For this review, take the finished solid that the model builds, in its own axes (mm). Coordinates: 2 decimals unless noted, no trailing zeros. Loops run counter-clockwise (first coordinate to the right, second up) from the corner with the lowest first, then second, coordinate; pieces in that order, holes last. Notation, with made-up numbers: M 59.25,79.5 L 80.25,79.5 A19 ccw 80.25,97.5 Z; hole C 28,19 d9. An arc over 180 degrees is marked long. Put each result on its own line as item: value.
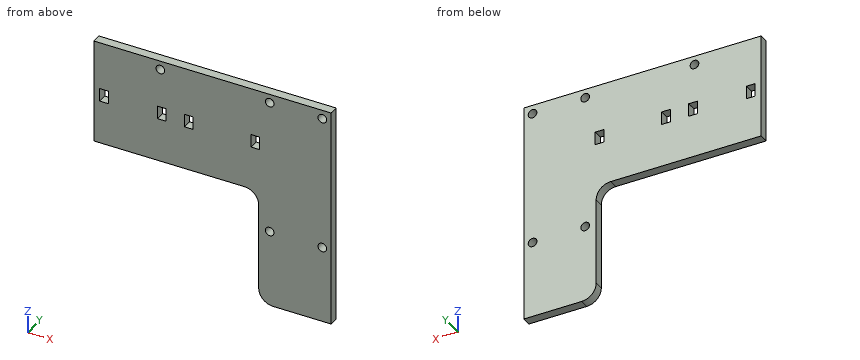
```python
from build123d import *

# Parameters (mm, degrees)
SKETCH1_W           = 25
SKETCH1_H           = 40
SKETCH1_W_2         = 82
SKETCH1_H_2         = 36
BOSS_EXTRUDE1_DEPTH = 3.175
CUT_EXTRUDE1_REACH  = 5.175
SKETCH2_R           = 1.5
SKETCH2_W           = 3
SKETCH2_H           = 4.5
FILLET1_R           = 5


with BuildPart() as part:
    # Sketch1 → Boss-Extrude1 (new body)
    with BuildSketch(Plane(origin=(0, 0, 0), x_dir=(1, 0, 0), z_dir=(0, 1, 0))):
        with Locations((69.5, 20)):
            Rectangle(SKETCH1_W, SKETCH1_H)
        with Locations((41, -18)):
            Rectangle(SKETCH1_W_2, SKETCH1_H_2)
    extrude(amount=BOSS_EXTRUDE1_DEPTH)

    # Sketch2 → Cut-Extrude1 (cut, up to next)
    with BuildSketch(Plane(origin=(0, 3.175, 0), x_dir=(1, 0, 0), z_dir=(0, 1, 0)), mode=Mode.PRIVATE) as cut_extrude1_sk1:
        with Locations((79, -33)):
            Circle(SKETCH2_R)
    cut_extrude1_tool1 = extrude(cut_extrude1_sk1.sketch, amount=-CUT_EXTRUDE1_REACH, mode=Mode.PRIVATE) & part.part
    add(cut_extrude1_tool1.solids().sort_by_distance((79, 3.175, 33))[0], mode=Mode.SUBTRACT)
    # Sketch2 → Cut-Extrude1 (cut, up to next)
    with BuildSketch(Plane(origin=(0, 3.175, 0), x_dir=(1, 0, 0), z_dir=(0, 1, 0)), mode=Mode.PRIVATE) as cut_extrude1_sk2:
        with Locations((60.8, -33)):
            Circle(SKETCH2_R)
    cut_extrude1_tool2 = extrude(cut_extrude1_sk2.sketch, amount=-CUT_EXTRUDE1_REACH, mode=Mode.PRIVATE) & part.part
    add(cut_extrude1_tool2.solids().sort_by_distance((60.8, 3.175, 33))[0], mode=Mode.SUBTRACT)
    # Sketch2 → Cut-Extrude1 (cut, up to next)
    with BuildSketch(Plane(origin=(0, 3.175, 0), x_dir=(1, 0, 0), z_dir=(0, 1, 0)), mode=Mode.PRIVATE) as cut_extrude1_sk3:
        with Locations((60.8, 13.4)):
            Circle(SKETCH2_R)
    cut_extrude1_tool3 = extrude(cut_extrude1_sk3.sketch, amount=-CUT_EXTRUDE1_REACH, mode=Mode.PRIVATE) & part.part
    add(cut_extrude1_tool3.solids().sort_by_distance((60.8, 3.175, -13.4))[0], mode=Mode.SUBTRACT)
    # Sketch2 → Cut-Extrude1 (cut, up to next)
    with BuildSketch(Plane(origin=(0, 3.175, 0), x_dir=(1, 0, 0), z_dir=(0, 1, 0)), mode=Mode.PRIVATE) as cut_extrude1_sk4:
        with Locations((79, 13.4)):
            Circle(SKETCH2_R)
    cut_extrude1_tool4 = extrude(cut_extrude1_sk4.sketch, amount=-CUT_EXTRUDE1_REACH, mode=Mode.PRIVATE) & part.part
    add(cut_extrude1_tool4.solids().sort_by_distance((79, 3.175, -13.4))[0], mode=Mode.SUBTRACT)
    # Sketch2 → Cut-Extrude1 (cut, up to next)
    with BuildSketch(Plane(origin=(0, 3.175, 0), x_dir=(1, 0, 0), z_dir=(0, 1, 0)), mode=Mode.PRIVATE) as cut_extrude1_sk5:
        with Locations((23, -33)):
            Circle(SKETCH2_R)
    cut_extrude1_tool5 = extrude(cut_extrude1_sk5.sketch, amount=-CUT_EXTRUDE1_REACH, mode=Mode.PRIVATE) & part.part
    add(cut_extrude1_tool5.solids().sort_by_distance((23, 3.175, 33))[0], mode=Mode.SUBTRACT)
    # Sketch2 → Cut-Extrude1 (cut, up to next)
    with BuildSketch(Plane(origin=(0, 3.175, 0), x_dir=(1, 0, 0), z_dir=(0, 1, 0)), mode=Mode.PRIVATE) as cut_extrude1_sk6:
        with Locations((32.85, -17.25)):
            Rectangle(SKETCH2_W, SKETCH2_H)
    cut_extrude1_tool6 = extrude(cut_extrude1_sk6.sketch, amount=-CUT_EXTRUDE1_REACH, mode=Mode.PRIVATE) & part.part
    add(cut_extrude1_tool6.solids().sort_by_distance((32.85, 3.175, 17.25))[0], mode=Mode.SUBTRACT)
    # Sketch2 → Cut-Extrude1 (cut, up to next)
    with BuildSketch(Plane(origin=(0, 3.175, 0), x_dir=(1, 0, 0), z_dir=(0, 1, 0)), mode=Mode.PRIVATE) as cut_extrude1_sk7:
        with Locations((55.85, -17.25)):
            Rectangle(SKETCH2_W, SKETCH2_H)
    cut_extrude1_tool7 = extrude(cut_extrude1_sk7.sketch, amount=-CUT_EXTRUDE1_REACH, mode=Mode.PRIVATE) & part.part
    add(cut_extrude1_tool7.solids().sort_by_distance((55.85, 3.175, 17.25))[0], mode=Mode.SUBTRACT)
    # Sketch2 → Cut-Extrude1 (cut, up to next)
    with BuildSketch(Plane(origin=(0, 3.175, 0), x_dir=(1, 0, 0), z_dir=(0, 1, 0)), mode=Mode.PRIVATE) as cut_extrude1_sk8:
        with Locations((3.5, -17.25)):
            Rectangle(SKETCH2_W, SKETCH2_H)
    cut_extrude1_tool8 = extrude(cut_extrude1_sk8.sketch, amount=-CUT_EXTRUDE1_REACH, mode=Mode.PRIVATE) & part.part
    add(cut_extrude1_tool8.solids().sort_by_distance((3.5, 3.175, 17.25))[0], mode=Mode.SUBTRACT)
    # Sketch2 → Cut-Extrude1 (cut, up to next)
    with BuildSketch(Plane(origin=(0, 3.175, 0), x_dir=(1, 0, 0), z_dir=(0, 1, 0)), mode=Mode.PRIVATE) as cut_extrude1_sk9:
        with Locations((23.5, -17.25)):
            Rectangle(SKETCH2_W, SKETCH2_H)
    cut_extrude1_tool9 = extrude(cut_extrude1_sk9.sketch, amount=-CUT_EXTRUDE1_REACH, mode=Mode.PRIVATE) & part.part
    add(cut_extrude1_tool9.solids().sort_by_distance((23.5, 3.175, 17.25))[0], mode=Mode.SUBTRACT)

    # Fillet1
    fillet1_edges = [part.edges().sort_by_distance(p)[0] for p in [
        (57, 1.5875, -40),
        (57, 1.5875, 0),
    ]]
    fillet(fillet1_edges, radius=FILLET1_R)


solid = part.part
```
(1) Add section A-A (z = 33). Write out the cut boundary in (x, y) (3 decimals).
Determined:
outline: M 0,0 L 21.5,0 L 21.5,3.175 L 0,3.175 Z; M 24.5,0 L 59.3,0 L 59.3,3.175 L 24.5,3.175 Z; M 62.3,0 L 77.5,0 L 77.5,3.175 L 62.3,3.175 Z; M 80.5,0 L 82,0 L 82,3.175 L 80.5,3.175 Z
(2) Wall thickness on line 1 along X through (y, z) = (2.45, 33); line 2 along Z through (x, y) = (79, 1.35); line 3 along X through (y, z) = (0.85, -13.4): over which ranges is each line inside the solid? List them lowest first. Write a range as [from, to].
Determined:
line 1: x = [0, 21.5], [24.5, 59.3], [62.3, 77.5], [80.5, 82]
line 2: z = [-40, -14.9], [-11.9, 31.5], [34.5, 36]
line 3: x = [57, 59.3], [62.3, 77.5], [80.5, 82]
(3) Add section D-D (y = 2.2). State how many separate pieces and enclosed holes the cut face has, plus the area to 3 significant figures.
Determined:
separate pieces: 1
enclosed holes: 9
area: 3,860 mm^2
(4) Add section C-C (z = -13.4). Write out the cut boundary in (x, y) (3 decimals).
Determined:
outline: M 57,0 L 59.3,0 L 59.3,3.175 L 57,3.175 Z; M 62.3,0 L 77.5,0 L 77.5,3.175 L 62.3,3.175 Z; M 80.5,0 L 82,0 L 82,3.175 L 80.5,3.175 Z
(5) Add section B-B (x = 79). Write out the cut boundary in (y, z) (3 decimals).
Determined:
outline: M 0,-40 L 3.175,-40 L 3.175,-14.9 L 0,-14.9 Z; M 0,-11.9 L 3.175,-11.9 L 3.175,31.5 L 0,31.5 Z; M 0,34.5 L 3.175,34.5 L 3.175,36 L 0,36 Z
(6) For pin 1 (1.8 mm diameter, centred on x = 60.8, z = 33, fed in from -Y); pin 2 (5 mm diameter, centred on x = 79, z = 33, fed in from +Y) (3 decimals); pin 3 (1 mm diameter, centred on y = 1, z = -17.5, fed in from -X); pin 4 (0.9 mm diameter, centred on x = 3.5, y = 1, fed in from -Z), all flat-tipped, find the tip position at first contact; note any pin that passes through.
Determined:
pin 1: passes through
pin 2: stops at y = 3.175
pin 3: stops at x = 57
pin 4: stops at z = 0
